Build history of the part. All positions in model axes, mm. Face numbers are marked on the shaded views. A direction names the side the tool comes from. Give positions to 0.01 mm unless a question says otherwise; leave off trailing zeros. Write each loop counter-clockwise with the first axis right and the second up, starting at its lowest first coordinate (ties: lowest second). Pieces come first, ordered by that corner, then holes.
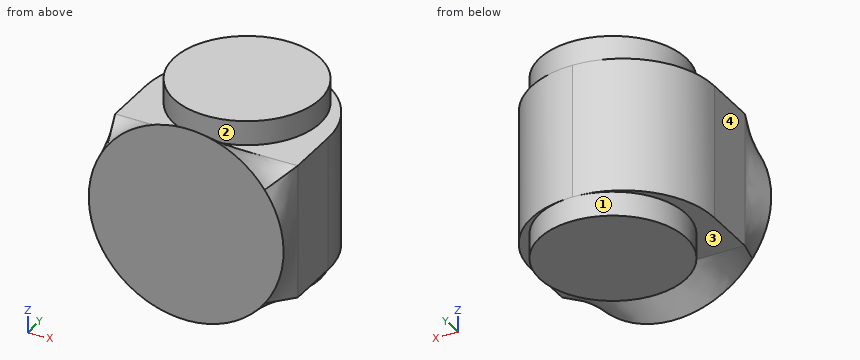
from build123d import *

# Parameters (mm, degrees)
SKIZZE4_W                       = 150
SKIZZE4_H                       = 110
AUFSATZ_LINEAR_AUSTRAGEN1_DEPTH = 120
SKIZZE5_R                       = 60
AUFSATZ_LINEAR_AUSTRAGEN2_DEPTH = 20
VERRUNDUNG1_R                   = 75


with BuildPart() as part:
    # Skizze1 for Ausformung1 → Ausformung1 section 0
    with BuildSketch(Plane(origin=(0, 0, 0), x_dir=(1, 0, 0), z_dir=(0, 1, 0))):
        with BuildLine():
            # circular arc as an exact rational Bezier (weights 1, cos(half-angle), 1)
            Bezier((-64.512399668, -47.30909309), (0, -135.280547185), (64.512399668, -47.30909309), weights=[1, 0.591363664, 1])
            Bezier((64.512399668, -47.30909309), (99.205734602, 0), (64.512399668, 47.30909309), weights=[1, 0.806404996, 1])
            Bezier((64.512399668, 47.30909309), (0, 135.280547185), (-64.512399668, 47.30909309), weights=[1, 0.591363664, 1])
            Bezier((-64.512399668, 47.30909309), (-99.205734602, 0), (-64.512399668, -47.30909309), weights=[1, 0.806404996, 1])
        make_face()
    # Skizze2 → Ausformung1 section 1
    with BuildSketch(Plane(origin=(0, 30, 0), x_dir=(1, 0, 0), z_dir=(0, 1, 0))):
        with BuildLine():
            Line((-75, -55), (75, -55))
            Line((75, -55), (75, 55))
            Line((75, 55), (-75, 55))
            Line((-75, 55), (-75, -55))
        make_face()
    loft()

    # Skizze4 → Aufsatz-Linear austragen1 (add)
    with BuildSketch(Plane(origin=(0, 30, 0), x_dir=(1, 0, 0), z_dir=(0, 1, 0))):
        Rectangle(SKIZZE4_W, SKIZZE4_H)
    extrude(amount=AUFSATZ_LINEAR_AUSTRAGEN1_DEPTH)

    # Skizze5 → Aufsatz-Linear austragen2 (add)
    with BuildSketch(Plane(origin=(-20, 0, 55), x_dir=(-1, 0, 0), z_dir=(0, 0, -1))):
        with Locations((-20, 90)):
            Circle(SKIZZE5_R)
    aufsatz_linear_austragen2 = extrude(amount=-AUFSATZ_LINEAR_AUSTRAGEN2_DEPTH)

    # Spiegeln1: Aufsatz-Linear austragen2 across plane
    add(aufsatz_linear_austragen2.mirror(Plane.XY))

    # Verrundung1
    # the kernel refuses this fillet: 75 mm, written as the material it takes off along each edge
    with BuildSketch(Plane(origin=(75, 150, 242.5), x_dir=(0, -1, 0), z_dir=(0, 0, -1))) as verrundung1_piece_1:
        with BuildLine():
            CenterArc((VERRUNDUNG1_R, VERRUNDUNG1_R), VERRUNDUNG1_R, 180, 90)
            Line((0, VERRUNDUNG1_R), (0, 0))
            Line((0, 0), (VERRUNDUNG1_R, 0))
        make_face()
    extrude(amount=485, mode=Mode.SUBTRACT)
    with BuildSketch(Plane(origin=(-75, 150, -242.5), x_dir=(1, 0, 0), z_dir=(0, 0, 1))) as verrundung1_piece_2:
        with BuildLine():
            CenterArc((VERRUNDUNG1_R, -VERRUNDUNG1_R), VERRUNDUNG1_R, 90, 90)
            Line((0, -VERRUNDUNG1_R), (0, 0))
            Line((0, 0), (VERRUNDUNG1_R, 0))
        make_face()
    extrude(amount=485, mode=Mode.SUBTRACT)


solid = part.part
(1) Saw through at A-A, the plane y = 62.5. List the corners of the cut face in (x, z).
(2) Drop flat-ended pins along their axis: pin 1 (12 mm diameter, centred on y = 65.5, z = -30, fed in from -X); pin 2 (10 mm diameter, centred on x = 48, z = -17.5, fed in from +Y); pin 3 (3 mm diameter, centred on x = -28, y = 75.5, fed in from +Z); pin 4 (8 mm diameter, centred on x = 13, z = 10, fed in from -Y). Give the stop position or say it passes through.
(3) Saw through at B-B, the plane y = 44. List the corners of the cut face in (x, z), plus the area to 3 significant figures.
(4) 3-axis set-ups, long thin cutter, end or side, ignore diameter. For the marked faces 1, 2, 3 and 4: which of +Z, -Z, +X, -X, +Y, -Y reach the whole face in a straight line?
(5) Probe line 1 (Z direction, x = 26.5, y = 84); line 2 (Z direction, x = 56.5, y = 124). List the from-to ranges inside material, lowest first.
Computed values:
1. outline: (-75, -55) - (-53.33, -55) - (-53.33, -75) - (53.33, -75) - (53.33, -55) - (75, -55) - (75, 55) - (53.33, 55) - (53.33, 75) - (-53.33, 75) - (-53.33, 55) - (-75, 55) - close
2. pin 1: stops at x = -75
2. pin 2: stops at y = 136.45
2. pin 3: stops at z = 75
2. pin 4: stops at y = 0
3. outline: (-75, -55) - (-38.52, -55) - (-38.52, -75) - (38.52, -75) - (38.52, -55) - (75, -55) - (75, 55) - (38.52, 55) - (38.52, 75) - (-38.52, 75) - (-38.52, 55) - (-75, 55) - close
3. area: 19,600 mm2
4. face 1: -Z
4. face 2: +Z
4. face 3: -Z, -X
4. face 4: +Z, -Z, -X, +Y
5. line 1: z = -75 to 75
5. line 2: z = -55 to 55
